The listing builds one solid part. Answer for the finished solid, in the listing's coordinates (mm). A direction names the side the tool comes from. Give positions to 0.01 mm unless a question says otherwise; leave off trailing zeros. Loops run counter-clockwise (first coordinate to the right, second up) from the corner with the lowest first, then second, coordinate; pieces in that order, holes last.
Item 1: Section A-A, the plane z = -2.54 is taken. Give the vertices of the cut face in (x, y).
Item 2: This flat-tipped pin is pushed along its axis until it touches: pin 1 Ø0.8 at (x, y) = (-7.5, 1) entering from -Z. Where does it stop, or does it pass through?
Item 3: Section D-D, the plane y = 0.6 is taken. Give the vertices of the cut face in (x, z).
Item 4: Section C-C, the plane z = -22 is taken. Give the vertices of the cut face in (x, y).
Item 5: A tool of negligible diameter and unlimited length cuts with its end or side. For faces 1 (the face through (-17, 1, -6.35)), 2 (the face through (-17, 1, 1.27)), 3 (the face through (0.102, 1, -3)), 4 (the face through (9.02, 1.25, -11.83)), from which of +Z, -Z, +X, -X, +Y, -Y can it reach the whole face along a straight path? Write none if from no direction.
Item 6: Section B-B, the plane x = -17 is taken. Give the vertices of the cut face in (y, z).
Item 7: Consider line 1 along X through (y, z) = (1.35, -2.54); line 2 along Z through (x, y) = (-16, 0.6); line 3 along Z through (x, y) = (12, 0.9). Determine where each line is inside the solid, lowest interval first.
from build123d import *

# Parameters (mm, degrees)
BOSS_EXTRUDE2_DEPTH = 2.54
SKETCH7_R           = 1.4986
SKETCH7_W           = 25.4
SKETCH7_H           = 5.08
CUT_EXTRUDE1_DEPTH  = 2.54


with BuildPart() as part:
    # Sketch1 → Boss-Extrude2 (new body)
    with BuildSketch(Plane(origin=(0, 0, 0), x_dir=(1, 0, 0), z_dir=(0, 1, 0))):
        Polygon((3.221868426, 6.029765094), (14.988277627, 17.796174295), (14.988277627, 29.226174295), (-4.295819053, 6.35), (-29.8704, 6.35), (-29.8704, -1.27), (-4.295819053, -1.27), (14.988277627, -24.146174295), (14.988277627, -12.716174295), (3.221868426, -0.949765094), align=None)
    extrude(amount=BOSS_EXTRUDE2_DEPTH)

    # Sketch7 → Cut-Extrude1 (cut)
    with BuildSketch(Plane(origin=(0, 2.54, 0), x_dir=(1, 0, 0), z_dir=(0, 1, 0))):
        with Locations(Location((-27.5844, 2.54, 0), (0, 0, 270))):
            Circle(SKETCH7_R)
        with Locations(Location((12.702277627, 22.713311162, 0), (0, 0, 270))):
            Circle(SKETCH7_R)
        with Locations(Location((12.622030753, 18.904156343, 0), (0, 0, 270))):
            Circle(SKETCH7_R)
        with Locations(Location((12.622030753, -13.824156343, 0), (0, 0, 90))):
            Circle(SKETCH7_R)
        with Locations(Location((12.702277627, -17.633311162, 0), (0, 0, 90))):
            Circle(SKETCH7_R)
        with Locations((-12.5984, 2.54)):
            Rectangle(SKETCH7_W, SKETCH7_H)
    extrude(amount=-CUT_EXTRUDE1_DEPTH, mode=Mode.SUBTRACT)


solid = part.part
Worked answers:
1. outline: (-29.87, 0) - (-29.08, 0) - (-29.08, 2.54) - (-29.87, 2.54) - close; (-26.09, 0) - (-25.3, 0) - (-25.3, 2.54) - (-26.09, 2.54) - close; (0.1, 0) - (3.22, 0) - (3.22, 2.54) - (0.1, 2.54) - close
2. pin 1: stops at z = -6.35
3. outline: (-29.87, -6.35) - (-4.3, -6.35) - (14.99, -29.23) - (14.99, -17.8) - (3.22, -6.03) - (3.22, 0.95) - (14.99, 12.72) - (14.99, 24.15) - (-4.3, 1.27) - (-29.87, 1.27) - close; hole circle Ø3 at (-27.58, -2.54); hole (-25.3, -5.08) - (0.1, -5.08) - (0.1, 0) - (-25.3, 0) - close; hole circle Ø3 at (12.62, -18.9); hole circle Ø3 at (12.62, 13.82); hole circle Ø3 at (12.7, -22.71); hole circle Ø3 at (12.7, 17.63)
4. outline: (8.9, 0) - (11.38, 0) - (11.38, 2.54) - (8.9, 2.54) - close; (14.02, 0) - (14.99, 0) - (14.99, 2.54) - (14.02, 2.54) - close
5. face 1: -Z, -X, +Y, -Y
5. face 2: +Z, -X, +Y, -Y
5. face 3: +Y, -Y
5. face 4: +X, +Y, -Y
6. outline: (0, -6.35) - (2.54, -6.35) - (2.54, -5.08) - (0, -5.08) - close; (0, 0) - (2.54, 0) - (2.54, 1.27) - (0, 1.27) - close
7. line 1: x = -29.87 to -29.08, -26.09 to -25.3, 0.1 to 3.22
7. line 2: z = -6.35 to -5.08, 0 to 1.27
7. line 3: z = -25.68 to -24.04, -21.39 to -20.27, -17.54 to -14.81, 9.73 to 12.46, 15.19 to 16.31, 18.96 to 20.6
